```python
from build123d import *

# Parameters (mm, degrees)
SKETCH1_R           = 7
SKETCH1_R_2         = 2.1
BOSS_EXTRUDE1_DEPTH = 5
SKETCH2_R           = 3.8
SKETCH2_R_2         = 2.1
BOSS_EXTRUDE2_DEPTH = 7.8
CHAMFER1_SIZE       = 0.4
CHAMFER1_SIZE2      = 0.399999869


with BuildPart() as part:
    # Sketch1 → Boss-Extrude1 (new body)
    with BuildSketch(Plane(origin=(0, 0, 0), x_dir=(1, 0, 0), z_dir=(0, 1, 0))):
        with Locations(Location((0, 0, 0), (0, 0, 270))):
            Circle(SKETCH1_R)
        with Locations(Location((0, 0, 0), (0, 0, 270))):
            Circle(SKETCH1_R_2, mode=Mode.SUBTRACT)
    extrude(amount=BOSS_EXTRUDE1_DEPTH)

    # Sketch2 → Boss-Extrude2 (add)
    with BuildSketch(Plane(origin=(0, 5, 0), x_dir=(1, 0, 0), z_dir=(0, 1, 0))):
        with Locations(Location((0, 0, 0), (0, 0, 270))):
            Circle(SKETCH2_R)
        with Locations(Location((0, 0, 0), (0, 0, 270))):
            Circle(SKETCH2_R_2, mode=Mode.SUBTRACT)
    extrude(amount=BOSS_EXTRUDE2_DEPTH)

    # Chamfer1
    chamfer1_edges = [part.edges().sort_by_distance(p)[0] for p in [
        (0, 0, -7),
    ]]
    chamfer1_side = [part.faces().sort_by_distance(p)[0] for p in [
        (0, 2.5, -7),
    ]]
    chamfer(chamfer1_edges, length=CHAMFER1_SIZE, length2=CHAMFER1_SIZE2, reference=chamfer1_side[0])


solid = part.part
```
Can you work these out from the model? Positions are in its coordinate system, mm. A direction names the side the tool comes from. Coordinates: 2 decimals unless noted, no trailing zeros. Order: outer loops, then holes, each group sorted by start corner. A loop starts at its lowest first (then second) coordinate and runs counter-clockwise, first axis right, second up.
1. Thinking about a two-plate mould opening in Z: for faces 3 (the face through (0.631, 6.31, 2.003)), 4 (the face through (-6.834, 2.668, -1.517)), 5 (the face through (-3, 5, 3)), which applies, +Z half, -Z half, draft (parallel to the pull), parting line (faces both ways), or undercut?
2. If we section it at C-C (y = 4.5): Please give me the cut outline in (x, z), then the cut area to 3 significant figures.
3. For faces 1 (the face through (2, 0, -2)), 2 (the face through (-1.46, 8.85, 3.51)), which set-ups out of +Z, -Z, +X, -X, +Y, -Y let a thin tool reach every point of the face, with its end or its side?
4. If we section it at A-A (x = 0): Please give me the cut outline in (y, z).
5. If we section it at D-D (y = 8): Please give me the cut outline in (x, z), then the cut area to 3 significant figures.
6. If we section it at B-B (z = 0): Please give me the cut outline in (x, y), then the cut area to 3 significant figures.
7. I'm going to push flat-ended pins straight in: pin 1 (1.5 mm diameter, centred on y = 5, z = -3, fed in from +X); pin 2 (2 mm diameter, centred on y = 7.5, z = 1, fed in from +X); pin 3 (2 mm diameter, centred on y = 7, z = 3.5, fed in from +X). Where does each tip first touch, or does it pass through?
8. I need wall thicknesses on line 1 (X direction, y = 3.25, z = 0); line 2 (X direction, y = 7, z = 0); line 3 (Y direction, x = -3.75, z = 4). Which ranges of each line are inside material? Lowest first, please.
Entries:
1. face 3: undercut
1. face 4: parting line
1. face 5: draft
2. outline: circle Ø14 at (0, 0); hole circle Ø4.2 at (0, 0)
2. area: 140 mm2
3. face 1: +Z, -Z, +X, -X, -Y
3. face 2: +Y
4. outline: (0, -6.6) - (0.4, -7) - (5, -7) - (5, -3.8) - (12.8, -3.8) - (12.8, -2.1) - (0, -2.1) - close; (0, 2.1) - (12.8, 2.1) - (12.8, 3.8) - (5, 3.8) - (5, 7) - (0.4, 7) - (0, 6.6) - close
5. outline: circle Ø7.6 at (0, 0); hole circle Ø4.2 at (0, 0)
5. area: 31.5 mm2
6. outline: (-7, 0.4) - (-6.6, 0) - (-2.1, 0) - (-2.1, 12.8) - (-3.8, 12.8) - (-3.8, 5) - (-7, 5) - close; (2.1, 0) - (6.6, 0) - (7, 0.4) - (7, 5) - (3.8, 5) - (3.8, 12.8) - (2.1, 12.8) - close
6. area: 75.4 mm2
7. pin 1: stops at x = 6.63
7. pin 2: stops at x = 3.8
7. pin 3: stops at x = 2.86
8. line 1: x = -7 to -2.1, 2.1 to 7
8. line 2: x = -3.8 to -2.1, 2.1 to 3.8
8. line 3: y = 0 to 5
